Design review of the part built by this model. Coordinates are the model's own, in mm. Give positions to 0.01 mm unless a question says otherwise; leave off trailing zeros. Loops run counter-clockwise (first coordinate to the right, second up) from the corner with the lowest first, then second, coordinate; pieces in that order, holes last. Notation, with made-up numbers: M 36,61.25 L 49,61.25 A14 ccw 49,69.25 Z; hole C 27.25,39 d3. An arc over 180 degrees is marked long. Use a Markdown table: item, result. Add a question column.
(1) Add section B-B, the plane y = -10. Give the boundary of the cut face in (x, z), then the cut area to 3 significant figures.
(2) For probe 1 along Y at (x, z) = (46.5, 1.8); probe 2 along X at (y, z) = (-10, 1.05); probe 3 along Y at (x, z) = (1, 0.55), list the stretches that pass through material, from the lowest coordinate up.
(3) Add section C-C, the plane z = 0.8. State how many separate pieces and enclosed holes the cut face has, then the cut area to 3 significant figures.
(4) Add section A-A, the plane x = 106.5. Give the boundary of the cut face in (y, z).
(5) Insertion check: pin 1 Ø1 at (y, z) = (-20, 3) entering from +X; pin 2 Ø4.5 at (x, y) = (31.63, -61.26) entering from -Z; pin 3 Ø3.5 at (x, y) = (-4.86, 6.15) entering from +Z; pin 4 Ø2 at (x, z) = (4, 2.5) entering from -Y. Each pin has a flat end and moves straight along its axis. Give the tip position at first contact, or say it passes through.
```python
from build123d import *

# Parameters (mm, degrees)
SKETCH1_R           = 2
SKETCH1_R_2         = 14.29
SKETCH1_R_3         = 2.499999953
SKETCH1_R_4         = 11
BOSS_EXTRUDE1_DEPTH = 4


with BuildPart() as part:
    # Sketch1 → Boss-Extrude1 (new body)
    with BuildSketch(Plane.XY):
        with BuildLine():
            Line((17.566132686, -48.57422294), (-4.85811184, -48.57422294))
            ThreePointArc((-4.85811184, -48.57422294), (-8.450214288, -47.086325388), (-9.93811184, -43.49422294))
            Line((-9.93811184, -43.49422294), (-10.688835244, 13.472862597))
            ThreePointArc((-10.688835244, 13.472862597), (-10.403338368, 14.676721118), (-9.582963432, 15.602879187))
            Line((-9.582963432, 15.602879187), (-6.619834827, 17.62947485))
            Line((-6.619834827, 17.62947485), (16.768305704, 33.625508255))
            Line((16.768305704, 33.625508255), (25.964523002, 39.915148892))
            ThreePointArc((25.964523002, 39.915148892), (27.966960045, 40.890333383), (30.165836856, 41.244846678))
            Line((30.165836856, 41.244846678), (171.657580351, 43.10945257))
            ThreePointArc((171.657580351, 43.10945257), (173.463278691, 42.389235045), (174.230829536, 40.603142807))
            Line((174.230829536, 40.603142807), (175.600950315, -63.36562536))
            ThreePointArc((175.600950315, -63.36562536), (174.869016667, -65.183273725), (173.061170841, -65.939095071))
            Line((173.061170841, -65.939095071), (66.523565599, -65.939095071))
            Line((66.523565599, -65.939095071), (31.633252021, -65.939095071))
            ThreePointArc((31.633252021, -65.939095071), (29.123552435, -65.208231246), (27.398652648, -63.244185761))
            Line((27.398652648, -63.244185761), (21.800732059, -51.26913225))
            ThreePointArc((21.800732059, -51.26913225), (20.075832272, -49.305086766), (17.566132686, -48.57422294))
        make_face()
        with Locations((-4.85811184, -43.49422294)):
            Circle(SKETCH1_R, mode=Mode.SUBTRACT)
        with Locations((101.811349412, -18.649052962)):
            Circle(SKETCH1_R_2, mode=Mode.SUBTRACT)
        with Locations((31.633252021, -61.264657987)):
            Circle(SKETCH1_R, mode=Mode.SUBTRACT)
        with Locations((30.266245989, 33.625508255)):
            Circle(SKETCH1_R, mode=Mode.SUBTRACT)
        with Locations((170.426367515, -60.775756941)):
            Circle(SKETCH1_R, mode=Mode.SUBTRACT)
        with Locations((161.513898191, 35.55251649)):
            Circle(SKETCH1_R, mode=Mode.SUBTRACT)
        with Locations((-4.85811184, 6.145317428)):
            Circle(SKETCH1_R, mode=Mode.SUBTRACT)
        with Locations((23.377209906, -42.310207828)):
            Circle(SKETCH1_R_3, mode=Mode.SUBTRACT)
        with Locations((23.377209906, -16.910207828)):
            Circle(SKETCH1_R_4, mode=Mode.SUBTRACT)
        with Locations((1.38016465, -29.610207828)):
            Circle(SKETCH1_R_3, mode=Mode.SUBTRACT)
        with Locations((1.38016465, -4.210207828)):
            Circle(SKETCH1_R_3, mode=Mode.SUBTRACT)
        with Locations((23.377209906, 8.489792172)):
            Circle(SKETCH1_R_3, mode=Mode.SUBTRACT)
        with Locations((45.374255162, -4.210207828)):
            Circle(SKETCH1_R_3, mode=Mode.SUBTRACT)
        with Locations((45.374255162, -29.610207828)):
            Circle(SKETCH1_R_3, mode=Mode.SUBTRACT)
    extrude(amount=BOSS_EXTRUDE1_DEPTH)


solid = part.part
```
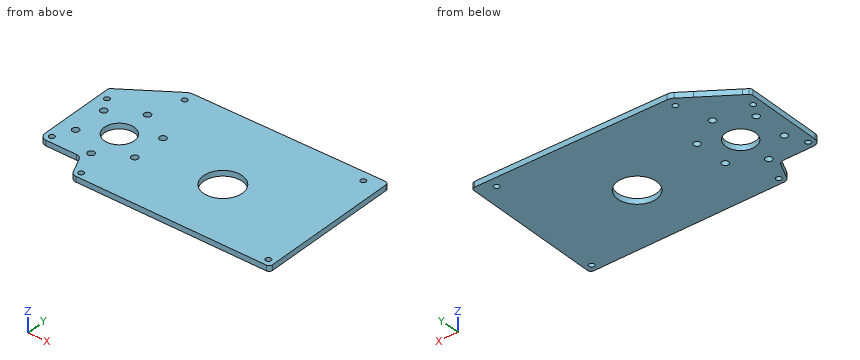
Established:
| question | item | result |
|---|---|---|
| 1 | outline | M -10.38,0 L 14.82,0 L 14.82,4 L -10.38,4 Z; M 31.94,0 L 90.44,0 L 90.44,4 L 31.94,4 Z; M 113.19,0 L 174.9,0 L 174.9,4 L 113.19,4 Z |
| 1 | area | 582 mm^2 |
| 2 | probe 1 | -65.94 to -31.84, -27.38 to -6.44, -1.98 to 41.46 |
| 2 | probe 2 | -10.38 to 14.82, 31.94 to 90.44, 113.19 to 174.9 |
| 2 | probe 3 | -48.57 to -32.08, -27.14 to -6.68, -1.74 to 22.84 |
| 3 | separate pieces | 1 |
| 3 | enclosed holes | 14 |
| 3 | area | 17,700 mm^2 |
| 4 | outline | M -65.94,0 L -32.15,0 L -32.15,4 L -65.94,4 Z; M -5.15,0 L 42.25,0 L 42.25,4 L -5.15,4 Z |
| 5 | pin 1 | x = 175.04 |
| 5 | pin 2 | z = 0 |
| 5 | pin 3 | through |
| 5 | pin 4 | y = -48.57 |
